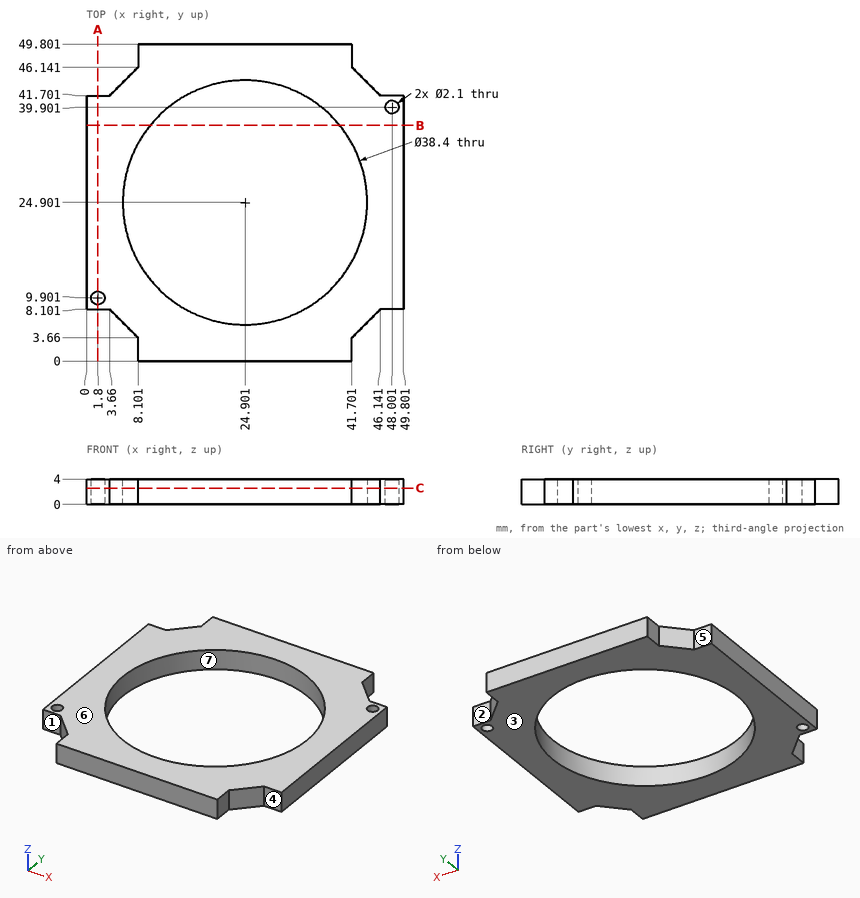
For this review, use the dimensioned drawing (mm, ordinates from the lowest corner) and the shaded views. A direction names the side the tool comes from. Give positions to 0.01 mm unless a question says otherwise; leave off trailing zeros. Order: outer loops, then holes, each group sorted by start corner. A loop starts at its lowest first (then second) coordinate and runs counter-clockwise, first axis right, second up. Notation, with made-up numbers: (-10.75, 5.5) - (29.25, 5.5) arc R30 cw to (29.25, 32.5) - close; hole circle Ø9 at (79.25, 79). An arc over 180 degrees is marked (long way). Write item = value, one per line. Start each with the question number.
Q1. We need section B-B on y = 37. State the section outline as (x, z) points.
Q2. We need section A-A on x = 1.8. State the section outline as (y, z) points, plus the area to 3 significant figures.
Q3. We need section C-C on z = 2.55. State the section outline as (x, y) points.
Q4. Clearance check with flat-ended pins moving along their axes: pin 1 Ø1.1 at (x, z) = (2, 1.5) entering from +Y; pin 2 Ø1.8 at (x, z) = (48, 1) entering from -Y; pin 3 Ø8 at (x, y) = (30.5, 37) entering from -Z; pin 4 Ø1.8 at (y, z) = (2.5, 2.5) entering from +X. State where each tip first meets the part, or that it passes through.
Q5. To check wall thickness, follow L1, parallel to Y at x = 1.8, z = 1; L2, parallel to X at y = 39.5, z = 0.95; L3, parallel to X at y = 40.5, z = 1.9 (1 decimal). State the ranges of each line that lie inside material, in increasing order. Write a range as from..to.
Q6. Mouldability with a two-part tool opening along Y and no side actions: class the marked faces 5, 6 and 7 as released by +Y, released by -Y, zero draft, split by the parting line, or undercut.
Q7. Tool access review of the marked faces 1, 2, 3 and 4: name each direction out of +Z, -Z, +X, -X, +Y, -Y from which nothing blocks a thin tool from reaching the whole face with its end or side.
Working result:
q1.outline = (0, 0) - (9.99, 0) - (9.99, 4) - (0, 4) - close; (39.81, 0) - (49.8, 0) - (49.8, 4) - (39.81, 4) - close
q2.outline = (8.1, 0) - (8.85, 0) - (8.85, 4) - (8.1, 4) - close; (10.95, 0) - (41.7, 0) - (41.7, 4) - (10.95, 4) - close
q2.area = 126 mm²
q3.outline = (0, 8.1) - (3.66, 8.1) - (8.1, 3.66) - (8.1, 0) - (41.7, 0) - (41.7, 3.66) - (46.14, 8.1) - (49.8, 8.1) - (49.8, 41.7) - (46.14, 41.7) - (41.7, 46.14) - (41.7, 49.8) - (8.1, 49.8) - (8.1, 46.14) - (3.66, 41.7) - (0, 41.7) - close; hole circle Ø2.1 at (1.8, 9.9); hole circle Ø38.4 at (24.9, 24.9); hole circle Ø2.1 at (48, 39.9)
q4.pin_1 = 41.7
q4.pin_2 = 8.1
q4.pin_3 = through
q4.pin_4 = 41.7
q5.L1 = 8.1..8.85, 10.95..41.7
q5.L2 = 0..12.43, 37.37..47.03, 48.97..49.8
q5.L3 = 0..13.7, 36.1..47.1, 48.9..49.8
q6.face_5 = released by +Y
q6.face_6 = zero draft
q6.face_7 = undercut
q7.face_1 = +Z, -Z, -X, -Y
q7.face_2 = +Z, -Z, +X, +Y
q7.face_3 = -Z, +X, -X, +Y, -Y
q7.face_4 = +Z, -Z, +X, -Y
